from build123d import *

# Parameters (mm, degrees)
BOSS_EXTRUDE1_DEPTH = 20
CUT_EXTRUDE1_DEPTH  = 21


with BuildPart() as part:
    # Sketch1 → Boss-Extrude1 (new body)
    with BuildSketch(Plane(origin=(0, 0, 0), x_dir=(0, 0, -1), z_dir=(1, 0, 0))):
        Polygon((0, 0), (0, 20), (3.175, 20), (3.175, 3.175), (20, 3.175), (20, 0), align=None)
    extrude(amount=BOSS_EXTRUDE1_DEPTH)

    # Sketch2 → Cut-Extrude1 (cut, through all)
    with BuildSketch(Plane(origin=(0, 0, 0), x_dir=(-1, 0, 0), z_dir=(0, -1, 0))):
        with BuildLine():
            Line((-7.75, 15.75), (-7.75, 5.75))
            ThreePointArc((-7.75, 5.75), (-10, 3.5), (-12.25, 5.75))
            Line((-12.25, 5.75), (-12.25, 15.75))
            ThreePointArc((-12.25, 15.75), (-10, 18), (-7.75, 15.75))
        make_face()
    extrude(amount=-CUT_EXTRUDE1_DEPTH, mode=Mode.SUBTRACT)


solid = part.part
Design review of the part built by this model. Coordinates are the model's own, in mm. A direction names the side the tool comes from. Coordinates: 2 decimals unless noted, no trailing zeros. Write each loop counter-clockwise with the first axis right and the second up, starting at its lowest first coordinate (ties: lowest second). Pieces come first, ordered by that corner, then holes. Notation, with made-up numbers: (76, -33.5) - (87, -33.5) arc R17 cw to (87, -8.5) - close; hole circle Ø5 at (-3.75, 32.25). An arc over 180 degrees is marked (long way). Use one line per item in the form item = value.
Q1. Consider section D-D (y = 17.75). Write out the cut boundary in (x, z) (3 decimals).
Taken from the geometry:
outline = (0, -3.175) - (20, -3.175) - (20, 0) - (0, 0) - close
Q2. Consider section B-B (z = -14.75). Write out the cut boundary in (x, y) (3 decimals), plus the area to 3 significant figures.
Taken from the geometry:
outline = (0, 0) - (7.75, 0) - (7.75, 3.175) - (0, 3.175) - close; (12.25, 0) - (20, 0) - (20, 3.175) - (12.25, 3.175) - close
area = 49.2 mm^2
Q3. Insertion check: pin 1 Ø8.5 at (x, z) = (8.5, -12.5) entering from +Y (3 decimals); pin 2 Ø10 at (y, z) = (15, -13) entering from +X; pin 3 Ø4 at (x, y) = (3.5, 7) entering from -Z (3 decimals). Each pin has a flat end and moves straight along its axis. Give the tip position at first contact, or say it passes through.
Taken from the geometry:
pin_1 = 3.175
pin_2 = through
pin_3 = -3.175
Q4. The part is to be moulded in two halves that separate along Z. For faces 1 (the flat face through (10, 2, -20)), 2 (the flat face through (12.25, 2, -11)), 3 (the flat face through (20, 6, -3)), 4 (the flat face through (7.75, 2, -11)), say which applies: +Z half, -Z half, draft (parallel to the pull), parting line (faces both ways), or undercut.
Taken from the geometry:
face_1 = -Z half
face_2 = undercut
face_3 = draft
face_4 = undercut
Q5. Consider section C-C (x = 4.75). Write out the cut boundary in (y, z) (3 decimals), plus the area to 3 significant figures.
Taken from the geometry:
outline = (0, -20) - (3.175, -20) - (3.175, -3.175) - (20, -3.175) - (20, 0) - (0, 0) - close
area = 117 mm^2
Q6. For probe 1 along Z at (x, y) = (12.5, 5) (3 decimals); probe 2 along Y at (x, z) = (13.5, -6.5) (3 decimals), list the stretches that pass through material, from the lowest coordinate up.
Taken from the geometry:
probe_1 = -3.175 to 0
probe_2 = 0 to 3.175
Q7. Consider section A-A (x = 10). Write out the cut boundary in (y, z) (3 decimals).
Taken from the geometry:
outline = (0, -20) - (3.175, -20) - (3.175, -18) - (0, -18) - close; (0, -3.5) - (3.175, -3.5) - (3.175, -3.175) - (20, -3.175) - (20, 0) - (0, 0) - close
Q8. Machinability: for faces 5 (the flat face through (10, 20, -2)), 6 (the cylindrical face through (10, 1.6, -3.5)), 7 (the flat face through (10, 12, -3.175)), which of the approach directions +Z, -Z, +X, -X, +Y, -Y give a long, thin tool a straight path to every point of the face, cutting with its end or side? Answer none if there is none.
Taken from the geometry:
face_5 = +Z, -Z, +X, -X, +Y
face_6 = +Y, -Y
face_7 = -Z, +X, -X, +Y
